Design review of the part built by this model. Coordinates are the model's own, in mm. Face numbers are marked on the shaded views. A direction names the side the tool comes from. Coordinates: 2 decimals unless noted, no trailing zeros. Loops run counter-clockwise (first coordinate to the right, second up) from the corner with the lowest first, then second, coordinate; pieces in that order, holes last. Notation, with made-up numbers: (31.25, 61) -> (57.25, 61) arc R32 ccw to (57.25, 87) -> close; hole circle Ø9 at (80, -17.75). An arc over 180 degrees is marked (long way). Use a Markdown table: item, result. Add a question column.
Q1. For probe 1 along X at (y, z) = (1.8, 9.5); probe 2 along Z at (x, y) = (0, 1.6); probe 3 along Z at (x, y) = (0, 4.05), list the stretches that pass through material, from the lowest coordinate up.
Q2. Clearance check with flat-ended pins moving along their axes: pin 1 Ø1 at (y, z) = (1.5, 1.5) entering from -X; pin 2 Ø0.8 at (y, z) = (5, -5.5) entering from +X; pin 3 Ø3.5 at (x, z) = (0, 0) entering from -Y. State where each tip first meets the part, or that it passes through.
Q3. For the marked faces 5, 6, 7 and 8, list the 3-axis set-ups (+Z, -Z, +X, -X, +Y, -Y) from which the entire face can be reached by the end or side of a thin tool; tool diameter is ignored.
Q4. Take a section at A-A on x = 0. Write out the cut boundary in (y, z).
Q5. Draft analysis for pull direction Z (two halves, no side actions). For the marked faces 1, 2, 3 and 4, state which applies: pulls with the +Z half, pulls with the -Z half, needs draft (parallel to the pull), parting line crosses it, or undercut.
Q6. Take a section at D-D on x = 5.25. Write out the cut boundary in (y, z), plus the area to 3 significant figures.
Q7. Take a section at C-C on z = -5.5. Write out the cut boundary in (x, y).
Q8. Take a section at B-B on z = 9.75. Write out the cut boundary in (x, y), plus the area to 3 significant figures.
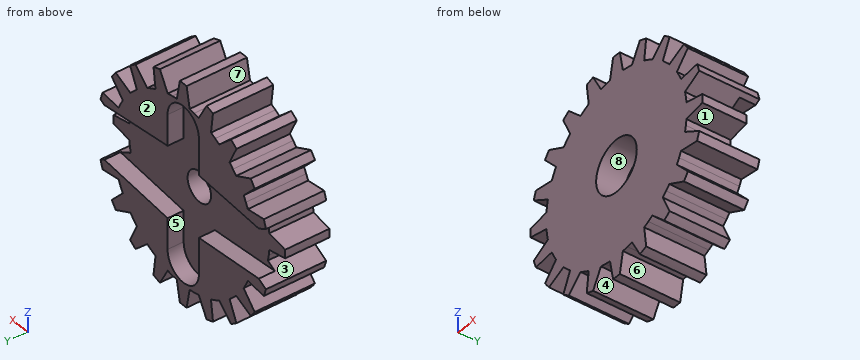
from build123d import *

# Parameters (mm, degrees)
SKETCH1_R           = 11
SKETCH1_R_2         = 1.5
BOSS_EXTRUDE1_DEPTH = 6
CUT_EXTRUDE1_DEPTH  = 6
CIRPATTERN1_COUNT   = 20
SKETCH3_R           = 1.25
CUT_EXTRUDE2_DEPTH  = 1.6
SKETCH4_R           = 2.6
CUT_EXTRUDE3_DEPTH  = 2.8


with BuildPart() as part:
    # Sketch1 → Boss-Extrude1 (new body)
    with BuildSketch(Plane(origin=(0, 0, 0), x_dir=(1, 0, 0), z_dir=(0, 1, 0))):
        Circle(SKETCH1_R)
        Circle(SKETCH1_R_2, mode=Mode.SUBTRACT)
    extrude(amount=BOSS_EXTRUDE1_DEPTH)

    # Sketch2 → Cut-Extrude1 (cut)
    with BuildSketch(Plane(origin=(0, 6, 0), x_dir=(1, 0, 0), z_dir=(0, 1, 0))):
        with BuildLine():
            Line((-0.823514568, 8.962244348), (-0.431857973, 10.991519399))
            ThreePointArc((-0.431857973, 10.991519399), (0, 11), (0.431857973, 10.991519399))
            Line((0.431857973, 10.991519399), (0.823514568, 8.962244348))
            ThreePointArc((0.823514568, 8.962244348), (1.116310063, 8.930501209), (1.407910185, 8.889195065))
            Line((1.407910185, 8.889195065), (2.683697474, 16.944198993))
            Line((2.683697474, 16.944198993), (-2.683697474, 16.944198993))
            Line((-2.683697474, 16.944198993), (-1.407910185, 8.889195065))
            ThreePointArc((-1.407910185, 8.889195065), (-1.116310063, 8.930501209), (-0.823514568, 8.962244348))
        make_face()
    cut_extrude1 = extrude(amount=-CUT_EXTRUDE1_DEPTH, mode=Mode.SUBTRACT)

    # CirPattern1: Cut-Extrude1 ×20 about axis
    cirpattern1_axis = Axis((0, 0, 0), (0, 1, 0))
    for i in range(1, CIRPATTERN1_COUNT):
        add(cut_extrude1.rotate(cirpattern1_axis, i * 360 / CIRPATTERN1_COUNT), mode=Mode.SUBTRACT)

    # Sketch3 → Cut-Extrude2 (cut)
    with BuildSketch(Plane(origin=(0, 6, 0), x_dir=(1, 0, 0), z_dir=(0, 1, 0))):
        with BuildLine():
            Line((-1.99882942, 6.681582528), (-1.99882942, 3.092373279))
            Line((-1.99882942, 3.092373279), (-15.754015296, 1.999995968))
            ThreePointArc((-15.754015296, 1.999995968), (-17.749999999, 0), (-15.754015296, -1.999995968))
            Line((-15.754015296, -1.999995968), (-1.99882942, -3.092373279))
            Line((-1.99882942, -3.092373279), (-1.99882942, -6.681582528))
            ThreePointArc((-1.99882942, -6.681582528), (0, -8.75), (1.99882942, -6.681582528))
            Line((1.99882942, -6.681582528), (1.99882942, -3.589755709))
            Line((1.99882942, -3.589755709), (15.756121614, -2.099991078))
            ThreePointArc((15.756121614, -2.099991078), (17.85, 0), (15.756121614, 2.099991078))
            Line((15.756121614, 2.099991078), (1.99882942, 3.589755709))
            Line((1.99882942, 3.589755709), (1.99882942, 6.681582528))
            ThreePointArc((1.99882942, 6.681582528), (0, 8.75), (-1.99882942, 6.681582528))
        make_face()
        Circle(SKETCH3_R, mode=Mode.SUBTRACT)
    extrude(amount=-CUT_EXTRUDE2_DEPTH, mode=Mode.SUBTRACT)

    # Sketch4 → Cut-Extrude3 (cut)
    with BuildSketch(Plane.XZ):
        Circle(SKETCH4_R)
    extrude(amount=-CUT_EXTRUDE3_DEPTH, mode=Mode.SUBTRACT)


solid = part.part
Answer list:
| question | item | result |
|---|---|---|
| 1 | probe 1 | -3.71 to -2.39, -0.72 to 0.72, 2.39 to 3.71 |
| 1 | probe 2 | -11 to -2.6, 2.6 to 11 |
| 1 | probe 3 | -11 to -1.5, 1.5 to 11 |
| 2 | pin 1 | x = -8.94 |
| 2 | pin 2 | x = 8.95 |
| 2 | pin 3 | y = 2.8 |
| 3 | face 5 | +Y |
| 3 | face 6 | -Z, +Y, -Y |
| 3 | face 7 | +Z, +Y, -Y |
| 3 | face 8 | -Y |
| 4 | outline | (0, -11) -> (6, -11) -> (6, -8.75) -> (4.4, -8.75) -> (4.4, -1.5) -> (2.8, -1.5) -> (2.8, -2.6) -> (0, -2.6) -> close; (0, 2.6) -> (2.8, 2.6) -> (2.8, 1.5) -> (4.4, 1.5) -> (4.4, 8.75) -> (6, 8.75) -> (6, 11) -> (0, 11) -> close |
| 5 | face 1 | undercut |
| 5 | face 2 | needs draft |
| 5 | face 3 | undercut |
| 5 | face 4 | pulls with the -Z half |
| 6 | outline | (0, -8.34) -> (6, -8.34) -> (6, -3.24) -> (4.4, -3.24) -> (4.4, 3.24) -> (6, 3.24) -> (6, 8.34) -> (0, 8.34) -> close |
| 6 | area | 89.7 mm² |
| 7 | outline | (-8.57, 0) -> (8.57, 0) -> (8.57, 6) -> (2, 6) -> (2, 4.4) -> (-2, 4.4) -> (-2, 6) -> (-8.57, 6) -> close |
| 8 | outline | (-3.74, 0) -> (-2.52, 0) -> (-2.52, 6) -> (-3.74, 6) -> close; (-0.67, 0) -> (0.67, 0) -> (0.67, 6) -> (-0.67, 6) -> close; (2.52, 0) -> (3.74, 0) -> (3.74, 6) -> (2.52, 6) -> close |
| 8 | area | 22.6 mm² |
